For this review, take the finished solid that the model builds, in its own axes (mm). A direction names the side the tool comes from. Coordinates: 2 decimals unless noted, no trailing zeros. Write each loop counter-clockwise with the first axis right and the second up, starting at its lowest first coordinate (ties: lowest second). Pieces come first, ordered by that corner, then holes.
Autodesk Inventor part; units mm, degrees
ref_plane "Work Plane1" through (0, 0, -218.75) normal (0, 0, 1) x (1, 0, 0)
ref_plane "YZ Plane" through (0, 0, 0) normal (1, 0, 0) x (0, 1, 0)
ref_plane "XZ Plane" through (0, 0, 0) normal (0, 1, 0) x (-1, 0, 0)
sketch "Sketch1" plane through (0, 0, 0) normal (0, 1, 0) x (-1, 0, 0)
  circle A0 centre (0, 0) radius 10
  line L0 (0, 0) -> (0, -437.5) construction
  line L1 (-30, 0) -> (-30, -437.5)
  line L2 (30, -437.5) -> (30, 0)
  arc A1 (30, 0) -> (-30, 0) centre (0, 0) ccw
  arc A2 (-30, -437.5) -> (30, -437.5) centre (0, -437.5) ccw
  circle A3 centre (0, -437.5) radius 10
  point P0 (0, -218.75)
  dimension "d0" = 20
  dimension "d1" = 437.5
  dimension "d2" = 20
  dimension "d3" = 30
extrude "Extrusion1" add sketch "Sketch1" along normal blind 8
sketch "Sketch2" plane through (0, 8, 0) normal (0, 1, 0) x (1, 0, 0)
  circle A0 centre (0, 0) radius 20
  circle A1 centre (0, 437.5) radius 10
  circle A2 centre (0, 437.5) radius 10
  circle A3 centre (0, 437.5) radius 20
  circle A4 centre (0, 0) radius 10
  dimension "d6" = 40
extrude "Extrusion2" cut sketch "Sketch2" against normal blind 4
sketch "Sketch3" plane through (0, 0, 0) normal (0, -1, 0) x (1, 0, 0)
  circle A0 centre (0, 0) radius 9
  circle A1 centre (0, 0) radius 11.5
  point P0 (0, 0)
  dimension "d9" = 23
extrude "Extrusion3" add sketch "Sketch3" along normal blind 2
sketch "Sketch4" plane through (0, 4, 0) normal (0, 1, 0) x (1, 0, 0)
  circle A0 centre (0, 0) radius 20
  circle A1 centre (0, 0) radius 10
  circle A2 centre (0, 437.5) radius 20
  circle A3 centre (0, 437.5) radius 10
  circle A4 centre (0, 0) radius 19
  circle A5 centre (0, 0) radius 11
  dimension "d12" = 38
  dimension "d13" = 22
extrude "Extrusion4" add sketch "Sketch4" along normal blind 15 contours A4
ref_plane "Work Plane1" through (0, 0, -218.75) normal (0, 0, 1) x (1, 0, 0)
mirror "Mirror1" about plane through (0, 0, -218.75) normal (0, 0, 1) of "Extrusion4"
move or copy body "Move Body1" bodies to move or copy 1 copy no rotation origin (0, 0, 0) rotation axis (0, 0, 1) rotation angle 90
properties part number "connecting rod" material "Steel, Mild"
Q1. Draft analysis for pull direction Y (two halves, no side actions). For faces 1 (the flat face through (-4, 2, 10)), 2 (the flat face through (-19, -8, -446)), 3 (the cylindrical face through (-3.944, -0.66, -467.493)), state which applies: +Y half, -Y half, draft (parallel to the pull), parting line (faces both ways), or undercut.
Ans:
face 1: undercut
face 2: draft
face 3: parting line
Q2. Add section A-A (x = -13). State the section outline as (y, z) points.
Ans:
outline: circle Ø38 at (0, -437.5); circle Ø38 at (0, 0); hole circle Ø22 at (0, -437.5); hole circle Ø22 at (0, 0)
Q3. For probe 1 along Z at (x, y) = (-1.9, 0); probe 2 along Z at (x, y) = (-15.25, 0); probe 3 along Z at (x, y) = (-13.5, -3.5), list the stretches that pass through material, from the lowest coordinate up.
Ans:
probe 1: z = -467.5 to -447.5, -427.5 to -10, 10 to 30
probe 2: z = -456.5 to -448.5, -426.5 to -418.5, -19 to -11, 11 to 19
probe 3: z = -456.17 to -447.93, -427.07 to -418.83, -18.67 to -10.43, 10.43 to 18.67
Q4. Add section B-B (y = 0). Give the number of separate pieces and of enclosed holes in the cut face, then the cut area to 3 significant figures.
Ans:
separate pieces: 3
enclosed holes: 0
area: 3,990 mm2
Q5. Clearance check with flat-ended pins moving along their axes: pin 1 Ø23 at (y, z) = (0, -437.5) entering from +X; pin 2 Ø4 at (y, z) = (21.5, -49.5) entering from -X; pin 3 Ø1.5 at (x, y) = (-9, 9) entering from -Z; pin 4 Ø24 at (y, z) = (0, -437.5) entering from -X. State where each tip first meets the part, or that it passes through.
Ans:
pin 1: stops at x = 0
pin 2: stops at x = -8
pin 3: stops at z = -454.62
pin 4: stops at x = -19
Q6. Add section C-C (z = -284). State the section outline as (x, y) points.
Ans:
outline: (-8, -30) - (0, -30) - (0, 30) - (-8, 30) - close
Q7. Tool access review of faces 4 (the flat face through (-4, 18, -430)), 5 (the cylindrical face through (0.986, -1.172, -8.923)): name each direction out of +Z, -Z, +X, -X, +Y, -Y from which nothing blocks a thin tool from reaching the whole face with its end or side.
Ans:
face 4: -X
face 5: +X, -X
